from build123d import *

# Parameters (mm, degrees)
SKETCH1_R           = 105
SKETCH1_R_2         = 80
BOSS_EXTRUDE1_DEPTH = 6.7
CUT_EXTRUDE3_DEPTH  = 6.7


with BuildPart() as part:
    # Sketch1 → Boss-Extrude1 (new body)
    with BuildSketch(Plane(origin=(0, 0, 0), x_dir=(1, 0, 0), z_dir=(0, 1, 0))):
        with Locations(Location((0, 0, 0), (0, 0, 270))):
            Circle(SKETCH1_R)
        with Locations(Location((0, 0, 0), (0, 0, 270))):
            Circle(SKETCH1_R_2, mode=Mode.SUBTRACT)
    extrude(amount=BOSS_EXTRUDE1_DEPTH)

    # Sketch2 → Cut-Extrude3 (cut)
    with BuildSketch(Plane(origin=(0, 6.7, 0), x_dir=(1, 0, 0), z_dir=(0, 1, 0))):
        with BuildLine():
            Line((88.131130638, -12.138217022), (74.442302871, -9.724507352))
            Line((74.442302871, -9.724507352), (73.278860081, -16.322719298))
            Line((73.278860081, -16.322719298), (86.967687848, -18.736428967))
            ThreePointArc((86.967687848, -18.736428967), (89.441724552, -22.269719556), (92.975015141, -19.795682851))
            Line((92.975015141, -19.795682851), (94.138457931, -13.197470906))
            ThreePointArc((94.138457931, -13.197470906), (91.664421227, -9.664180317), (88.131130638, -12.138217022))
        make_face()
        with BuildLine():
            Line((75.314658396, 47.351185103), (63.276905284, 40.401185103))
            Line((63.276905284, 40.401185103), (66.626905284, 34.598814897))
            Line((66.626905284, 34.598814897), (78.664658396, 41.548814897))
            ThreePointArc((78.664658396, 41.548814897), (82.831035878, 40.432437416), (83.94741336, 44.598814897))
            Line((83.94741336, 44.598814897), (80.59741336, 50.401185103))
            ThreePointArc((80.59741336, 50.401185103), (76.431035878, 51.517562584), (75.314658396, 47.351185103))
        make_face()
        with BuildLine():
            Line((59.710067386, -65.948012501), (50.775319611, -55.299994741))
            Line((50.775319611, -55.299994741), (45.642821842, -59.606671726))
            Line((45.642821842, -59.606671726), (54.577569617, -70.254689486))
            ThreePointArc((54.577569617, -70.254689486), (54.201636275, -74.551627247), (58.498574036, -74.927560589))
            Line((58.498574036, -74.927560589), (63.631071805, -70.620883604))
            ThreePointArc((63.631071805, -70.620883604), (64.007005147, -66.323945843), (59.710067386, -65.948012501))
        make_face()
        with BuildLine():
            Line((3.35, -88.9), (3.35, -75))
            Line((3.35, -75), (-3.35, -75))
            Line((-3.35, -75), (-3.35, -88.9))
            ThreePointArc((-3.35, -88.9), (-6.4, -91.95), (-3.35, -95))
            Line((-3.35, -95), (3.35, -95))
            ThreePointArc((3.35, -95), (6.4, -91.95), (3.35, -88.9))
        make_face()
        with BuildLine():
            Line((-54.577569617, -70.254689486), (-45.642821842, -59.606671726))
            Line((-45.642821842, -59.606671726), (-50.775319611, -55.299994741))
            Line((-50.775319611, -55.299994741), (-59.710067386, -65.948012501))
            ThreePointArc((-59.710067386, -65.948012501), (-64.007005147, -66.323945843), (-63.631071805, -70.620883604))
            Line((-63.631071805, -70.620883604), (-58.498574036, -74.927560589))
            ThreePointArc((-58.498574036, -74.927560589), (-54.201636275, -74.551627247), (-54.577569617, -70.254689486))
        make_face()
        with BuildLine():
            Line((-86.967687848, -18.736428967), (-73.278860081, -16.322719298))
            Line((-73.278860081, -16.322719298), (-74.442302871, -9.724507352))
            Line((-74.442302871, -9.724507352), (-88.131130638, -12.138217022))
            ThreePointArc((-88.131130638, -12.138217022), (-91.664421227, -9.664180317), (-94.138457931, -13.197470906))
            Line((-94.138457931, -13.197470906), (-92.975015141, -19.795682851))
            ThreePointArc((-92.975015141, -19.795682851), (-89.441724552, -22.269719556), (-86.967687848, -18.736428967))
        make_face()
        with BuildLine():
            Line((-78.664658396, 41.548814897), (-66.626905284, 34.598814897))
            Line((-66.626905284, 34.598814897), (-63.276905284, 40.401185103))
            Line((-63.276905284, 40.401185103), (-75.314658396, 47.351185103))
            ThreePointArc((-75.314658396, 47.351185103), (-76.431035878, 51.517562584), (-80.59741336, 50.401185103))
            Line((-80.59741336, 50.401185103), (-83.94741336, 44.598814897))
            ThreePointArc((-83.94741336, 44.598814897), (-82.831035878, 40.432437416), (-78.664658396, 41.548814897))
        make_face()
    extrude(amount=-CUT_EXTRUDE3_DEPTH, mode=Mode.SUBTRACT)


solid = part.part
Check sheet for the modelled part. Datum: model origin and axes. Units: mm. Give positions to 0.01 mm unless a question says otherwise; leave off trailing zeros. Write each loop counter-clockwise with the first axis right and the second up, starting at its lowest first coordinate (ties: lowest second). Pieces come first, ordered by that corner, then holes. Notation, with made-up numbers: (27, -36.5) -> (34, -36.5) arc R9 cw to (34, -27.5) -> close; hole circle Ø9 at (76, 43). An arc over 180 degrees is marked (long way). Write item = value, one per line.
Item 1: Sectioned sample at C-C on z = -83. Record the boundary of the cut face in (x, y), and give its area (3 significant figures).
Output:
outline = (-64.31, 0) -> (64.31, 0) -> (64.31, 6.7) -> (-64.31, 6.7) -> close
area = 862 mm^2
Item 2: Sectioned sample at A-A on x = 0. Record the boundary of the cut face in (y, z).
Output:
outline = (0, -105) -> (6.7, -105) -> (6.7, -80) -> (0, -80) -> close; (0, 95) -> (6.7, 95) -> (6.7, 105) -> (0, 105) -> close
Item 3: Scan lines: probe 1 along X at (y, z) = (2.75, 70); probe 2 along Z at (x, y) = (61, 1); probe 3 along Z at (x, y) = (0.5, 4.5). Record each from-to range of solid material in increasing order. Write a range as from..to.
Output:
probe_1 = -78.26..-64.19, -54.36..-38.73, 38.73..54.36, 64.19..78.26
probe_2 = -85.46..-51.76, 51.76..65.31, 72.83..85.46
probe_3 = -105..-80, 95..105
Item 4: Release check for a two-part mould opening along Z. For faces 1 (the flat face through (-77, 6.7, -24)), 2 (the cylindrical face through (31.54, 3.3, 100.15)), 3 (the flat face through (3.35, 3, 84)) record: +Z half, -Z half, draft (parallel to the pull), parting line (faces both ways), or undercut.
Output:
face_1 = draft
face_2 = parting line
face_3 = undercut
Item 5: Gauge pin test, flat ends, axial feed: pin 1 (2 mm diameter, centred on y = 3, z = 86.5, fed in from +X); pin 2 (2 mm diameter, centred on y = 2, z = 83, fed in from -X); pin 3 (4 mm diameter, centred on y = 1, z = 51.5, fed in from -X). Record the tip position at first contact, or that the pin passes through.
Output:
pin_1 = 60.95
pin_2 = -65.58
pin_3 = -92.6
Item 6: Sectioned sample at B-B on z = 0. Record the boundary of the cut face in (x, y), and give its area (3 significant figures).
Output:
outline = (-105, 0) -> (-80, 0) -> (-80, 6.7) -> (-105, 6.7) -> close; (80, 0) -> (105, 0) -> (105, 6.7) -> (80, 6.7) -> close
area = 335 mm^2
